Part model, mm, in its own coordinate system. Coordinates: 2 decimals unless noted, no trailing zeros. Order: outer loops, then holes, each group sorted by start corner. A loop starts at its lowest first (then second) coordinate and runs counter-clockwise, first axis right, second up. Notation, with made-up numbers: (-37, 11) - (4, 11) arc R12 ccw to (4, 25) - close; hole circle Ø1 at (5.5, 70.25). An arc over 180 degrees is marked (long way). Use a Markdown table: item, result. Add a question column.
1) Wall check: L1, parallel to X at y = 6.2, z = -75 (3 decimals); L2, parallel to X at y = 6.5, z = -58; L3, parallel to X at y = 4, z = -47.5. Give the ranges that are in metal, low to high. Write a range as [from, to].
2) Drop flat-ended pins along their axis: P1, Ø25, axis at x = 15, z = -29.82, coming from the +Y side; P2, Ø2.5, axis at x = 71, z = -40, coming from the +Y side. Give the stop position or say it passes through.
3) Saw through at A-A on x = 89.5. List the corners of the cut face in (y, z), then the cut area to 3 significant figures.
4) Saw through at B-B on z = -57.5. List the corners of the cut face in (x, y).
5) Saw through at C-C on z = -20.5. List the corners of the cut face in (x, y) (3 decimals), then the cut area to 3 significant figures.
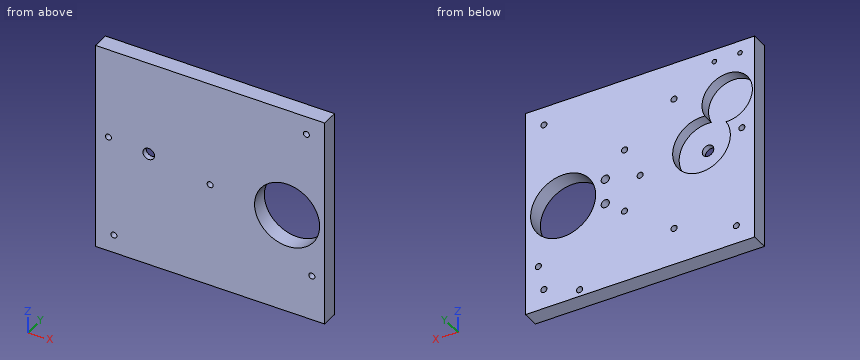
```python
from build123d import *

# Parameters (mm, degrees)
SKETCH1_W                 = 125
SKETCH1_H                 = 115
TOP_BASE_DEPTH            = 9
SKETCH5_R                 = 15.75
SKETCH5_R_2               = 13.75
GEARS_EXTRUDE_CUT_DEPTH   = 6
SKETCH7_R                 = 3.15
KEY_EXTRUDE_CUT_DEPTH     = 171.091152033
SKETCH8_R                 = 17.75
THUMB_EXTRUDE_CUT_DEPTH   = 171.091152033
SKETCH9_R                 = 1.675
SKETCH9_R_2               = 2.25
MOUNT_HOLES_DEPTH         = 5
M3X0_5_TAPPED_HOLE1_D     = 2.5
M3X0_5_TAPPED_HOLE1_DEPTH = 7.5
M3X0_5_TAPPED_HOLE1_TIP   = 0.751075774
M4X0_7_TAPPED_HOLE1_D     = 3.3
M4X0_7_TAPPED_HOLE1_DEPTH = 10.1
M4X0_7_TAPPED_HOLE1_TIP   = 0.991420021


with BuildPart() as part:
    # Sketch1 → Top_Base (new body)
    with BuildSketch(Plane(origin=(0, 0, 0), x_dir=(1, 0, 0), z_dir=(0, 1, 0))):
        with Locations((62.5, 57.5)):
            Rectangle(SKETCH1_W, SKETCH1_H)
    extrude(amount=TOP_BASE_DEPTH)

    # Sketch5 → Gears_Extrude_Cut (cut)
    with BuildSketch(Plane(origin=(0, 9, 0), x_dir=(1, 0, 0), z_dir=(0, 1, 0))):
        with Locations((29.01540546, 51.79347369)):
            Circle(SKETCH5_R)
        with Locations((15, 29.820255536)):
            Circle(SKETCH5_R_2)
    extrude(amount=-GEARS_EXTRUDE_CUT_DEPTH, mode=Mode.SUBTRACT)

    # Sketch7 → Key_Extrude_Cut (cut, through all)
    with BuildSketch(Plane(origin=(0, 9, 0), x_dir=(1, 0, 0), z_dir=(0, 1, 0))):
        with Locations(Location((29.01540546, 51.79347369, 0), (0, 0, 270))):
            Circle(SKETCH7_R)
    extrude(amount=-KEY_EXTRUDE_CUT_DEPTH, mode=Mode.SUBTRACT)

    # Sketch8 → Thumb_Extrude_Cut (cut, through all)
    with BuildSketch(Plane(origin=(0, 9, 0), x_dir=(1, 0, 0), z_dir=(0, 1, 0))):
        with Locations(Location((104.5, 60, 0), (0, 0, 270))):
            Circle(SKETCH8_R)
    extrude(amount=-THUMB_EXTRUDE_CUT_DEPTH, mode=Mode.SUBTRACT)

    # Sketch9 → Mount_Holes (cut)
    with BuildSketch(Plane(origin=(0, 9, 0), x_dir=(1, 0, 0), z_dir=(0, 1, 0))):
        with Locations(Location((71, 75, 0), (0, 0, 270))):
            Circle(SKETCH9_R)
        with Locations(Location((44, 94.5, 0), (0, 0, 270))):
            Circle(SKETCH9_R)
        with Locations(Location((81.5, 67, 0), (0, 0, 270))):
            Circle(SKETCH9_R_2)
        with Locations(Location((95.5, 111.25, 0), (0, 0, 270))):
            Circle(SKETCH9_R)
        with Locations(Location((115, 104.25, 0), (0, 0, 270))):
            Circle(SKETCH9_R)
        with Locations(Location((71, 40, 0), (0, 0, 90))):
            Circle(SKETCH9_R)
        with Locations(Location((44, 20.5, 0), (0, 0, 90))):
            Circle(SKETCH9_R)
        with Locations(Location((81.5, 53, 0), (0, 0, 90))):
            Circle(SKETCH9_R_2)
    extrude(amount=-MOUNT_HOLES_DEPTH, mode=Mode.SUBTRACT)

    # M3x0.5 Tapped Hole1
    with Locations(Plane(origin=(8, 9, -6.820255536), x_dir=(0, 0, 1), z_dir=(0, 1, 0))):
        with Locations((0, 0), (0, 14)):
            Hole(M3X0_5_TAPPED_HOLE1_D / 2, depth=M3X0_5_TAPPED_HOLE1_DEPTH)
            with Locations((0, 0, -(M3X0_5_TAPPED_HOLE1_DEPTH + M3X0_5_TAPPED_HOLE1_TIP / 2))):  # 118° drill point
                Cone(0, M3X0_5_TAPPED_HOLE1_D / 2, M3X0_5_TAPPED_HOLE1_TIP, mode=Mode.SUBTRACT)

    # M4x0.7 Tapped Hole1
    with Locations(Plane(origin=(10, 9, -105), x_dir=(0, 0, 1), z_dir=(0, 1, 0))):
        with Locations((0, 0), (15, 108), (95, 105), (55, -3), (47.5, 52.5)):
            Hole(M4X0_7_TAPPED_HOLE1_D / 2, depth=M4X0_7_TAPPED_HOLE1_DEPTH)
            with Locations((0, 0, -(M4X0_7_TAPPED_HOLE1_DEPTH + M4X0_7_TAPPED_HOLE1_TIP / 2))):  # 118° drill point
                Cone(0, M4X0_7_TAPPED_HOLE1_D / 2, M4X0_7_TAPPED_HOLE1_TIP, mode=Mode.SUBTRACT)


solid = part.part
```
Results are:
| question | item | result |
|---|---|---|
| 1 | L1 | [0, 69.325], [72.675, 95.01], [113.99, 125] |
| 1 | L2 | [0, 14.54], [43.49, 60.93], [64.07, 86.86], [122.14, 125] |
| 1 | L3 | [0, 13.86], [44.17, 91.9], [117.1, 125] |
| 2 | P1 | y = 3 |
| 2 | P2 | y = 4 |
| 3 | outline | (0, -115) - (9, -115) - (9, -69.49) - (0, -69.49) - close; (0, -50.51) - (9, -50.51) - (9, 0) - (0, 0) - close |
| 3 | area | 864 mm2 |
| 4 | outline | (0, 0) - (60.85, 0) - (60.85, 9) - (43.7, 9) - (43.7, 3) - (14.34, 3) - (14.34, 9) - (0, 9) - close; (64.15, 0) - (86.93, 0) - (86.93, 9) - (64.15, 9) - close; (122.07, 0) - (125, 0) - (125, 9) - (122.07, 9) - close |
| 5 | outline | (0, 0) - (125, 0) - (125, 9) - (45.675, 9) - (45.675, 4) - (42.325, 4) - (42.325, 9) - (25.109, 9) - (25.109, 3) - (4.891, 3) - (4.891, 9) - (0, 9) - close |
| 5 | area | 987 mm2 |
